from build123d import *

# Parameters (mm, degrees)
SKETCH_1_W                   = 196
SKETCH_1_H                   = 246
EXTRUDE_1_DEPTH              = 22
HOLE_WIZARD_M101_D           = 11
HOLE_WIZARD_M101_CBORE_D     = 18
HOLE_WIZARD_M101_CBORE_DEPTH = 13
HOLE_WIZARD_M221_D           = 26


with BuildPart() as part:
    # Эскиз1 → Бобышка-Вытянуть1 (new body)
    with BuildSketch(Plane.XY.offset(22)):
        Rectangle(SKETCH_1_W, SKETCH_1_H)
    extrude(amount=-EXTRUDE_1_DEPTH)

    # Цековка для  болта с шестигранной головкой M101 (through all)
    with Locations(Plane.XY.offset(22)):
        with Locations((50, 77), (50, -77), (-50, 77), (-50, -77)):
            CounterBoreHole(HOLE_WIZARD_M101_D / 2, HOLE_WIZARD_M101_CBORE_D / 2, HOLE_WIZARD_M101_CBORE_DEPTH)

    # Отверстие с зазором M221 (through all)
    with Locations(Plane.XY.offset(22)):
        with Locations((76, 77), (76, -77), (-76, -77), (-76, 77)):
            Hole(HOLE_WIZARD_M221_D / 2)


solid = part.part
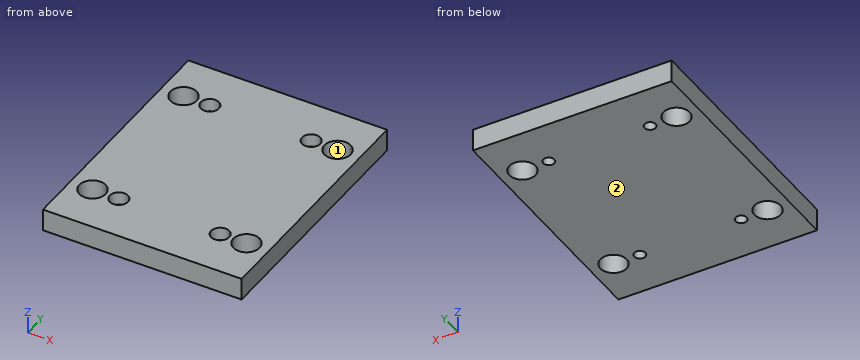
Could you check a few things on this model? Use its own coordinates, in mm. Face numbers are marked on the shaded views. Coordinates: 2 decimals unless noted, no trailing zeros. Loops run counter-clockwise (first coordinate to the right, second up) from the corner with the lowest first, then second, coordinate; pieces in that order, holes last.
1. Imagine slicing it at D-D (x = -76). Please give me the cut outline in (y, z), and give its area (3 significant figures).
2. Imagine slicing it at B-B (y = -77). Please give me the cut outline in (x, z).
3. For P1, Ø16, axis at x = -50, y = -77, coming from the +Z side; P2, Ø20, axis at x = 50, y = 77.5, coming from the +Z side, each with a flat end and sliding along its axis, tell me the tip position at first contact or that it passes through.
4. We'd pull the mould along X, two halves only. Please class the marked faces 1 and 2: released by +X, released by -X, zero draft, split by the parting line, or undercut.
5. Imagine slicing it at A-A (x = 50). Please give me the cut outline in (y, z).
6. I need wall thicknesses on L1, parallel to Y at x = -76, z = 10; L2, parallel to Y at x = -50, z = 15.5; L3, parallel to X at y = 82, z = 14.75. Which ranges of each line are inside material? Lowest first, please.
7. Imagine slicing it at C-C (z = 2.75). Give the number of separate pieces and of enclosed holes in the cut face, and give its area (3 significant figures).
Computed values:
1. outline: (-123, 0) - (-90, 0) - (-90, 22) - (-123, 22) - close; (-64, 0) - (64, 0) - (64, 22) - (-64, 22) - close; (90, 0) - (123, 0) - (123, 22) - (90, 22) - close
1. area: 4,270 mm2
2. outline: (-98, 0) - (-89, 0) - (-89, 22) - (-98, 22) - close; (-63, 0) - (-55.5, 0) - (-55.5, 9) - (-59, 9) - (-59, 22) - (-63, 22) - close; (-44.5, 0) - (44.5, 0) - (44.5, 9) - (41, 9) - (41, 22) - (-41, 22) - (-41, 9) - (-44.5, 9) - close; (55.5, 0) - (63, 0) - (63, 22) - (59, 22) - (59, 9) - (55.5, 9) - close; (89, 0) - (98, 0) - (98, 22) - (89, 22) - close
3. P1: stops at z = 9
3. P2: stops at z = 22
4. face 1: undercut
4. face 2: zero draft
5. outline: (-123, 0) - (-82.5, 0) - (-82.5, 9) - (-86, 9) - (-86, 22) - (-123, 22) - close; (-71.5, 0) - (71.5, 0) - (71.5, 9) - (68, 9) - (68, 22) - (-68, 22) - (-68, 9) - (-71.5, 9) - close; (82.5, 0) - (123, 0) - (123, 22) - (86, 22) - (86, 9) - (82.5, 9) - close
6. L1: y = -123 to -90, -64 to 64, 90 to 123
6. L2: y = -123 to -86, -68 to 68, 86 to 123
6. L3: x = -98 to -88, -64 to -57.48, -42.52 to 42.52, 57.48 to 64, 88 to 98
7. separate pieces: 1
7. enclosed holes: 8
7. area: 45,700 mm2
